```python
from build123d import *

# Parameters (mm, degrees)
SKETCH_1_W          = 140
SKETCH_1_H          = 70
SKETCH_1_R          = 1.6
SKETCH_1_R_2        = 5
EXTRUDE_1_DEPTH     = 3
SKETCH_2_W          = 29
SKETCH_2_H          = 23
SKETCH_2_W_2        = 52
SKETCH_2_H_2        = 20
CUT_EXTRUDE_1_DEPTH = 79.319856997
FILLET_1_R          = 3
CHAMFER_1_SIZE      = 8
SKETCH_3_R          = 2.1
SKETCH_3_R_2        = 1.6
CUT_EXTRUDE_2_DEPTH = 79.319856997


with BuildPart() as part:
    # 草图1 → 凸台-拉伸1 (new body)
    with BuildSketch(Plane.XY):
        Rectangle(SKETCH_1_W, SKETCH_1_H)
        with Locations((-25, 5)):
            Circle(SKETCH_1_R, mode=Mode.SUBTRACT)
        with Locations((25, 5)):
            Circle(SKETCH_1_R, mode=Mode.SUBTRACT)
        with Locations((-25, -5)):
            Circle(SKETCH_1_R, mode=Mode.SUBTRACT)
        with Locations((25, -5)):
            Circle(SKETCH_1_R, mode=Mode.SUBTRACT)
        Circle(SKETCH_1_R_2, mode=Mode.SUBTRACT)
    extrude(amount=EXTRUDE_1_DEPTH)

    # 草图2 → 切除-拉伸1 (cut, through all)
    with BuildSketch(Plane.XY.offset(3)):
        with Locations((-47.5, 15.5)):
            Rectangle(SKETCH_2_W, SKETCH_2_H)
        with Locations((-47.5, -15.5)):
            Rectangle(SKETCH_2_W, SKETCH_2_H)
        with Locations((47.5, -15.5)):
            Rectangle(SKETCH_2_W, SKETCH_2_H)
        with Locations((47.5, 15.5)):
            Rectangle(SKETCH_2_W, SKETCH_2_H)
        with Locations((0, 18)):
            Rectangle(SKETCH_2_W_2, SKETCH_2_H_2)
        with Locations((0, -18)):
            Rectangle(SKETCH_2_W_2, SKETCH_2_H_2)
    extrude(amount=-CUT_EXTRUDE_1_DEPTH, mode=Mode.SUBTRACT)

    # 圆角1
    fillet_1_edges = [part.edges().sort_by_distance(p)[0] for p in [
        (-62, -27, 1.5),
        (-62, -4, 1.5),
        (-33, -4, 1.5),
        (-33, -27, 1.5),
        (26, 28, 1.5),
        (26, 8, 1.5),
        (-26, 8, 1.5),
        (-26, 28, 1.5),
        (62, -4, 1.5),
        (62, -27, 1.5),
        (33, -27, 1.5),
        (33, -4, 1.5),
        (62, 27, 1.5),
        (62, 4, 1.5),
        (33, 4, 1.5),
        (33, 27, 1.5),
        (26, -8, 1.5),
        (26, -28, 1.5),
        (-26, -28, 1.5),
        (-26, -8, 1.5),
        (-62, 4, 1.5),
        (-62, 27, 1.5),
        (-33, 27, 1.5),
        (-33, 4, 1.5),
    ]]
    fillet(fillet_1_edges, radius=FILLET_1_R)

    # 倒角1
    chamfer_1_edges = [part.edges().sort_by_distance(p)[0] for p in [
        (-70, 35, 1.5),
        (70, 35, 1.5),
        (70, -35, 1.5),
        (-70, -35, 1.5),
    ]]
    chamfer(chamfer_1_edges, length=CHAMFER_1_SIZE)

    # 草图3 → 切除-拉伸2 (cut, through all)
    with BuildSketch(Plane.XY.offset(3)):
        with Locations((-46.5, 0)):
            Circle(SKETCH_3_R)
        with Locations((46.5, 0)):
            Circle(SKETCH_3_R)
        with Locations((-57.5, 0)):
            Circle(SKETCH_3_R_2)
        with Locations(Location((57.5, 0, 0), (0, 0, 180))):
            Circle(SKETCH_3_R_2)
        with Locations(Location((35.5, 0, 0), (0, 0, 180))):
            Circle(SKETCH_3_R_2)
        with Locations((-65.5, 0)):
            Circle(SKETCH_3_R_2)
        with Locations(Location((65.5, 0, 0), (0, 0, 180))):
            Circle(SKETCH_3_R_2)
    extrude(amount=-CUT_EXTRUDE_2_DEPTH, mode=Mode.SUBTRACT)


solid = part.part
```
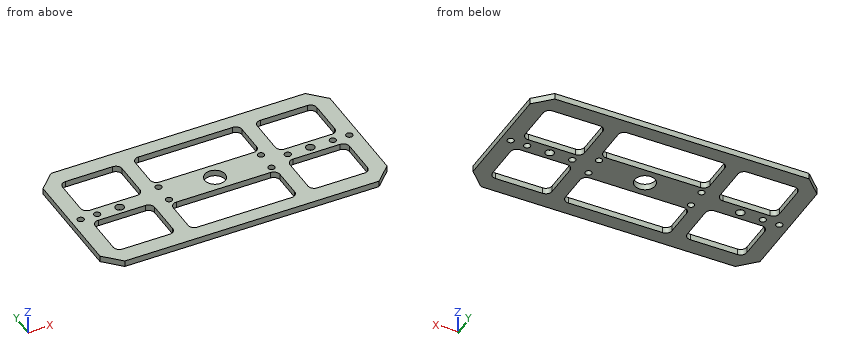
Verification items for the finished model (mm, model axes). Coordinates: 2 decimals unless noted, no trailing zeros. Loops run counter-clockwise (first coordinate to the right, second up) from the corner with the lowest first, then second, coordinate; pieces in that order, holes last. Notation, with made-up numbers: (-21.5, 83) - (5.5, 83) arc R17 ccw to (5.5, 114) - close; hole circle Ø10 at (-21, -15.5). An arc over 180 degrees is marked (long way). Answer as a JSON object with one key per item and string values.
(1) Cross-section at A-A, the plane x = 12.5. Record the boundary of the cut face in (y, z).
Response:
{"outline": "(-35, 0) - (-28, 0) - (-28, 3) - (-35, 3) - close; (-8, 0) - (8, 0) - (8, 3) - (-8, 3) - close; (28, 0) - (35, 0) - (35, 3) - (28, 3) - close"}
(2) Scan lines: line 1 along Y through (x, z) = (-46.5, 2.35); line 2 along Y through (x, z) = (-12.5, 1.05); line 3 along X through (y, z) = (12, 1.5). Record each from-to range of solid material in increasing order.
Response:
{"line 1": "y = -35 to -27, -4 to -2.1, 2.1 to 4, 27 to 35", "line 2": "y = -35 to -28, -8 to 8, 28 to 35", "line 3": "x = -70 to -62, -33 to -26, 26 to 33, 62 to 70"}
(3) Cross-section at C-C, the plane x = 46.5. Record the boundary of the cut face in (y, z), then the cut area to 3 significant figures.
Response:
{"outline": "(-35, 0) - (-27, 0) - (-27, 3) - (-35, 3) - close; (-4, 0) - (-2.1, 0) - (-2.1, 3) - (-4, 3) - close; (2.1, 0) - (4, 0) - (4, 3) - (2.1, 3) - close; (27, 0) - (35, 0) - (35, 3) - (27, 3) - close", "area": "59.4 mm²"}
(4) Cross-section at B-B, the plane y = 22.5. Record the boundary of the cut face in (x, z).
Response:
{"outline": "(-70, 0) - (-62, 0) - (-62, 3) - (-70, 3) - close; (-33, 0) - (-26, 0) - (-26, 3) - (-33, 3) - close; (26, 0) - (33, 0) - (33, 3) - (26, 3) - close; (62, 0) - (70, 0) - (70, 3) - (62, 3) - close"}
(5) Cross-section at D-D, the plane x = -65.5. Record the boundary of the cut face in (y, z).
Response:
{"outline": "(-31.5, 0) - (-1.6, 0) - (-1.6, 3) - (-31.5, 3) - close; (1.6, 0) - (31.5, 0) - (31.5, 3) - (1.6, 3) - close"}
